```python
from build123d import *

# Parameters (mm, degrees)
CUT_EXTRUDE1_DEPTH = 10


with BuildPart() as part:
    # Sketch1 → Revolve2 (revolve)
    with BuildSketch(Plane.XY, mode=Mode.PRIVATE) as revolve2_sk:
        with BuildLine():
            Line((8, 8), (8, -8))
            Line((8, -8), (14, -8))
            Line((14, -8), (14, -5))
            Line((14, -5), (184, -5))
            Line((184, -5), (184, -8))
            Line((184, -8), (190, -8))
            Line((190, -8), (190, -4))
            ThreePointArc((190, -4), (186, 0), (190, 4))
            Line((190, 4), (190, 8))
            Line((190, 8), (184, 8))
            Line((184, 8), (184, 5))
            Line((184, 5), (14, 5))
            Line((14, 5), (14, 8))
            Line((14, 8), (14, 18))
            Line((14, 18), (8, 18))
            Line((8, 18), (8, 8))
        make_face()
    revolve(revolve2_sk.sketch.rotate(Axis((0, 60.317614973, 0), (0, -1, 0)), 90), axis=Axis((0, 60.317614973, 0), (0, -1, 0)))

    # Sketch2 → Cut-Extrude1 (cut)
    with BuildSketch(Plane(origin=(0, 5, 0), x_dir=(1, 0, 0), z_dir=(0, 1, 0))):
        with BuildLine():
            Line((14, 14), (14, 173.435867109))
            ThreePointArc((14, 173.435867109), (123.036579926, 123.036579926), (173.435867109, 14))
            Line((173.435867109, 14), (14, 14))
        make_face()
        with BuildLine():
            Line((-173.435867109, -14), (-14, -14))
            Line((-14, -14), (-14, -173.435867109))
            ThreePointArc((-14, -173.435867109), (-123.036579926, -123.036579926), (-173.435867109, -14))
        make_face()
        with BuildLine():
            Line((-14, 14), (-14, 173.435867109))
            ThreePointArc((-14, 173.435867109), (-123.036579926, 123.036579926), (-173.435867109, 14))
            Line((-173.435867109, 14), (-14, 14))
        make_face()
        with BuildLine():
            Line((14, -14), (173.435867109, -14))
            ThreePointArc((173.435867109, -14), (123.036579926, -123.036579926), (14, -173.435867109))
            Line((14, -173.435867109), (14, -14))
        make_face()
    extrude(amount=-CUT_EXTRUDE1_DEPTH, mode=Mode.SUBTRACT)


solid = part.part
```
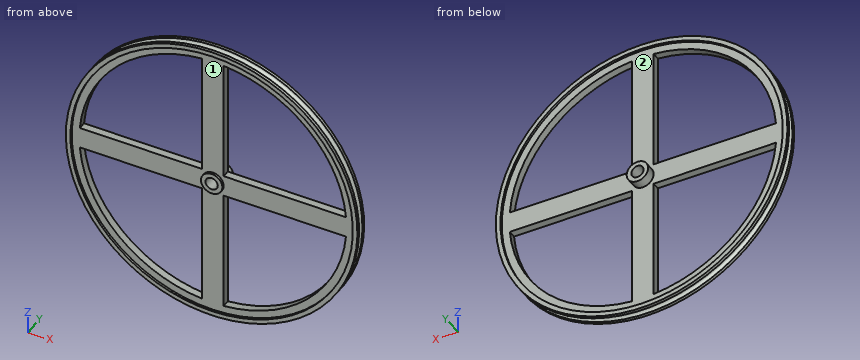
The listing builds one solid part. Answer for the finished solid, in the listing's coordinates (mm). Face numbers are marked on the shaded views. A direction names the side the tool comes from. Round coordinates to 2 decimals unless told otherwise and drop trailing zeros. Write each loop counter-clockwise with the first axis right and the second up, starting at its lowest first coordinate (ties: lowest second). Pieces come first, ordered by that corner, then holes. Notation, with made-up numbers: (84.5, -35.5) -> (120.5, -35.5) arc R9 cw to (120.5, -21.5) -> close; hole circle Ø8 at (-28.5, 33). An arc over 180 degrees is marked (long way). Write item = value, one per line.
1) Section A-A on z = 0 is taken. Write down the section's boundary in (x, y), plus the area to 3 significant figures.
Check values:
outline = (-190, -8) -> (-184, -8) -> (-184, -5) -> (-14, -5) -> (-14, -8) -> (-8, -8) -> (-8, 18) -> (-14, 18) -> (-14, 5) -> (-184, 5) -> (-184, 8) -> (-190, 8) -> (-190, 4) arc R4 cw to (-190, -4) -> close; (8, -8) -> (14, -8) -> (14, -5) -> (184, -5) -> (184, -8) -> (190, -8) -> (190, -4) arc R4 cw to (190, 4) -> (190, 8) -> (184, 8) -> (184, 5) -> (14, 5) -> (14, 18) -> (8, 18) -> close
area = 3,850 mm²
2) Straight lines are drawn through the part: line 1 along X through (y, z) = (5.85, 0); line 2 along Z through (x, y) = (-95, -4.75); line 3 along X through (y, z) = (3.25, 77.5). For each, find the intervals that lie inside material, in ascending order. Write a range as [from, to].
Check values:
line_1 = [-190, -184], [-14, -8], [8, 14], [184, 190]
line_2 = [-164.54, -145.78], [-14, 14], [145.78, 164.54]
line_3 = [-170.92, -155.79], [-14, 14], [155.79, 170.92]
3) Section B-B on x = 0 is taken. Write down the section's boundary in (y, z).
Check values:
outline = (-8, -190) -> (-4, -190) arc R4 cw to (4, -190) -> (8, -190) -> (8, -184) -> (5, -184) -> (5, -14) -> (18, -14) -> (18, -8) -> (-8, -8) -> (-8, -14) -> (-5, -14) -> (-5, -184) -> (-8, -184) -> close; (-8, 8) -> (18, 8) -> (18, 14) -> (5, 14) -> (5, 184) -> (8, 184) -> (8, 190) -> (4, 190) arc R4 cw to (-4, 190) -> (-8, 190) -> (-8, 184) -> (-5, 184) -> (-5, 14) -> (-8, 14) -> close
4) Section C-C on x = -102 is taken. Give the number of separate pieces and of enclosed holes in the cut face, plus the area to 3 significant figures.
Check values:
separate_pieces = 3
enclosed_holes = 0
area = 693 mm²
5) Which of the six approach directions +Z, -Z, +X, -X, +Y, -Y give full straight-line access (tool end or side, diameter ignored) to the marked faces 1 and 2?
Check values:
face_1 = -Y
face_2 = +Y
6) Given pin 1 (4 mm diameter, centred on x = -136.5, y = 6.5, fed in from +Z); pin 2 (8 mm diameter, centred on x = -47.5, y = 7.5, fed in from +Z); pin 3 (11 mm diameter, centred on x = -101, y = 0, fed in from -Z), each flat-ended and moving along its own axis, determine where each tip first touches the part or whether it passes through.
Check values:
pin_1 = 134.2
pin_2 = 184.95
pin_3 = -163.24
